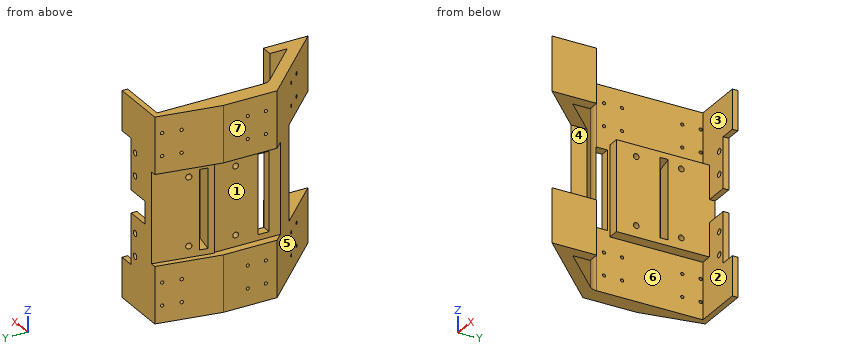
from build123d import *

# Parameters (mm, degrees)
BOSS_EXTRUDE2_DEPTH = 180
SKETCH2_R           = 2.5
CUT_EXTRUDE1_DEPTH  = 180
SKETCH3_W           = 10
SKETCH3_H           = 82.5
CUT_EXTRUDE2_DEPTH  = 35
BOSS_EXTRUDE3_DEPTH = 34
CUT_EXTRUDE3_DEPTH  = 205.147272565
SKETCH6_R           = 2.5
CUT_EXTRUDE4_DEPTH  = 34
CUT_EXTRUDE5_DEPTH  = 5
SKETCH8_W           = 80
SKETCH8_H           = 62.155508182
CUT_EXTRUDE8_DEPTH  = 7
CUT_EXTRUDE9_DEPTH  = 205.147272565
SKETCH11_W          = 10
SKETCH11_H          = 35
BOSS_EXTRUDE4_DEPTH = 5
SKETCH12_W          = 15
SKETCH12_H          = 82.5
CUT_EXTRUDE11_DEPTH = 10
SKETCH10_R          = 1.4
CUT_EXTRUDE10_DEPTH = 18
SKETCH14_R          = 1.4
CUT_EXTRUDE12_DEPTH = 211.50767784
BOSS_EXTRUDE5_DEPTH = 14
SKETCH16_R          = 1.5
CUT_EXTRUDE13_DEPTH = 219.238688301
SKETCH17_W          = 70
SKETCH17_H          = 7
CUT_EXTRUDE14_DEPTH = 210.498896517
SKETCH18_W          = 70
SKETCH18_H          = 10
CUT_EXTRUDE15_DEPTH = 209.444279941
BOSS_EXTRUDE6_DEPTH = 48
FILLET1_R           = 10


# Read off the part's stored shape, not the designer's step: Boss-Extrude2
with BuildPart() as part:
    # Boss-Extrude2 outline → Boss-Extrude2 (new body)
    with BuildSketch(Plane.XY):
        Polygon((-25, 32.5), (-25, -32.5), (-15, -87.5), (25, -87.5), (25, -82.5), (0, -82.5), (0, 82.5), (25, 82.5), (25, 87.5), (-15, 87.5), align=None)
    extrude(amount=BOSS_EXTRUDE2_DEPTH)

    # Sketch2 → Cut-Extrude1 (cut)
    with BuildSketch(Plane(origin=(0, 87.5, 0), x_dir=(1, 0, 0), z_dir=(0, 1, 0))):
        Polygon((25, -35), (21, -35), (21, -80), (0, -80), (0, -100), (21, -100), (21, -145), (25, -145), align=None)
        with Locations(Location((15, -45, 0), (0, 0, 270))):
            Circle(SKETCH2_R)
        with Locations(Location((15, -65, 0), (0, 0, 270))):
            Circle(SKETCH2_R)
        with Locations(Location((15, -115, 0), (0, 0, 270))):
            Circle(SKETCH2_R)
        with Locations(Location((15, -135, 0), (0, 0, 270))):
            Circle(SKETCH2_R)
    extrude(amount=-CUT_EXTRUDE1_DEPTH, mode=Mode.SUBTRACT)

    # Sketch3 → Cut-Extrude2 (cut)
    with BuildSketch(Plane.XY.offset(180)):
        with Locations((-5, 41.25)):
            Rectangle(SKETCH3_W, SKETCH3_H)
    cut_extrude2 = extrude(amount=-CUT_EXTRUDE2_DEPTH, mode=Mode.SUBTRACT)

    # Mirror1: Cut-Extrude2 across plane
    add(cut_extrude2.mirror(Plane.XY.offset(90)), mode=Mode.SUBTRACT)

    # Sketch4 → Boss-Extrude3 (add)
    with BuildSketch(Plane.XY.offset(180)):
        Polygon((-10, 0), (40.247470675, -50.247470675), (40.247470675, -80.498358966), (-25, -15.250888291), align=None)
    boss_extrude3 = extrude(amount=-BOSS_EXTRUDE3_DEPTH)

    # Mirror2: Boss-Extrude3 across plane
    add(boss_extrude3.mirror(Plane.XY.offset(90)))

    # Sketch5 → Cut-Extrude3 (cut, through all)
    with BuildSketch(Plane.XY.offset(180)):
        Polygon((0, 0), (-10, 0), (0, -10), align=None)
        Polygon((0, -40.250888291), (-25, -15.250888291), (-25, -32.5), (-15, -87.5), (25, -87.5), (25, -82.5), (0, -82.5), align=None)
    extrude(amount=-CUT_EXTRUDE3_DEPTH, mode=Mode.SUBTRACT)

    # Sketch6 → Cut-Extrude4 (cut)
    with BuildSketch(Plane(origin=(0, 0, 0), x_dir=(0, 0, -1), z_dir=(1, 0, 0))):
        with Locations(Location((-120, 57.5, 0), (0, 0, 90))):
            Circle(SKETCH6_R)
        with Locations(Location((-60, 57.5, 0), (0, 0, 90))):
            Circle(SKETCH6_R)
        with Locations(Location((-120, 17.5, 0), (0, 0, 90))):
            Circle(SKETCH6_R)
        with Locations(Location((-60, 17.5, 0), (0, 0, 90))):
            Circle(SKETCH6_R)
    extrude(amount=-CUT_EXTRUDE4_DEPTH, mode=Mode.SUBTRACT)

    # Sketch7 → Cut-Extrude5 (cut)
    with BuildSketch(Plane(origin=(-29.92, 5.44, 0), x_dir=(0, 0, 1), z_dir=(-0.9838699100999075, 0.17888543819998307, 0))):
        Polygon((50, 83.405335561), (50, 27.503636123), (130, 27.503636123), (130, 85.782619375), (130, 90.970472455), (50, 90.970472455), align=None)
    extrude(amount=-CUT_EXTRUDE5_DEPTH, mode=Mode.SUBTRACT)

    # Sketch8 → Cut-Extrude8 (cut)
    with BuildSketch(Plane.ZY.offset(25)):
        with Locations((90, 5.923338625)):
            Rectangle(SKETCH8_W, SKETCH8_H)
    extrude(amount=-CUT_EXTRUDE8_DEPTH, mode=Mode.SUBTRACT)

    # Sketch9 → Cut-Extrude9 (cut, through all)
    with BuildSketch(Plane.XY.offset(180)):
        Polygon((-10, 0), (40.247470675, -50.247470675), (40.247470675, -66.356223342), (-10, -16.108752667), align=None)
    extrude(amount=-CUT_EXTRUDE9_DEPTH, mode=Mode.SUBTRACT)

    # Sketch11 → Boss-Extrude4 (add)
    with BuildSketch(Plane(origin=(0, 87.5, 0), x_dir=(1, 0, 0), z_dir=(0, 1, 0))):
        with Locations((30, -17.5)):
            Rectangle(SKETCH11_W, SKETCH11_H)
        with Locations((30, -162.5)):
            Rectangle(SKETCH11_W, SKETCH11_H)
    extrude(amount=-BOSS_EXTRUDE4_DEPTH)

    # Sketch12 → Cut-Extrude11 (cut)
    with BuildSketch(Plane(origin=(0, 0, 0), x_dir=(0, 0, -1), z_dir=(1, 0, 0))):
        with Locations((-137.5, 41.25)):
            Rectangle(SKETCH12_W, SKETCH12_H)
        with Locations((-42.5, 41.25)):
            Rectangle(SKETCH12_W, SKETCH12_H)
    extrude(amount=-CUT_EXTRUDE11_DEPTH, mode=Mode.SUBTRACT)

    # Sketch10 → Cut-Extrude10 (cut)
    with BuildSketch(Plane(origin=(-29.92, 5.44, 0), x_dir=(0, 0, 1), z_dir=(-0.9838699100999075, 0.17888543819998307, 0))):
        with Locations(Location((165, 77.405335561, 0), (0, 0, 270))):
            Circle(SKETCH10_R)
        with Locations(Location((145, 77.405335561, 0), (0, 0, 270))):
            Circle(SKETCH10_R)
        with Locations(Location((145, 61.405335561, 0), (0, 0, 270))):
            Circle(SKETCH10_R)
        with Locations(Location((165, 61.405335561, 0), (0, 0, 270))):
            Circle(SKETCH10_R)
    cut_extrude10 = extrude(amount=-CUT_EXTRUDE10_DEPTH, mode=Mode.SUBTRACT)

    # Mirror3: Cut-Extrude10 across plane
    add(cut_extrude10.mirror(Plane.XY.offset(90)), mode=Mode.SUBTRACT)

    # Sketch14 → Cut-Extrude12 (cut, through all)
    with BuildSketch(Plane.ZY.offset(25)):
        with Locations((165, -5.250888291)):
            Circle(SKETCH14_R)
        with Locations((145, -5.250888291)):
            Circle(SKETCH14_R)
        with Locations((145, 10.749111709)):
            Circle(SKETCH14_R)
        with Locations((165, 10.749111709)):
            Circle(SKETCH14_R)
    cut_extrude12 = extrude(amount=-CUT_EXTRUDE12_DEPTH, mode=Mode.SUBTRACT)

    # Sketch15 → Boss-Extrude5 (add)
    with BuildSketch(Plane(origin=(0, 0, 146), x_dir=(-1, 0, 0), z_dir=(0, 0, -1))):
        Polygon((0, -40.250888291), (0, -26.108752667), (-40.247470675, -66.356223342), (-40.247470675, -80.498358966), align=None)
    boss_extrude5 = extrude(amount=BOSS_EXTRUDE5_DEPTH)

    # Mirror4: Boss-Extrude5 across plane
    add(boss_extrude5.mirror(Plane.XY.offset(90)))

    # Mirror5: Cut-Extrude12 across plane
    add(cut_extrude12.mirror(Plane.XY.offset(90)), mode=Mode.SUBTRACT)

    # Sketch16 → Cut-Extrude13 (cut, through all)
    with BuildSketch(Plane(origin=(-20.125444145, -20.125444145, 0), x_dir=(0, 0, 1), z_dir=(-0.7071067811865476, -0.7071067811865476, 0))):
        with Locations(Location((165, -35.380194939, 0), (0, 0, 270))):
            Circle(SKETCH16_R)
        with Locations(Location((145, -35.380194939, 0), (0, 0, 270))):
            Circle(SKETCH16_R)
        with Locations(Location((145, -51.380194939, 0), (0, 0, 270))):
            Circle(SKETCH16_R)
        with Locations(Location((165, -51.380194939, 0), (0, 0, 270))):
            Circle(SKETCH16_R)
    cut_extrude13 = extrude(amount=-CUT_EXTRUDE13_DEPTH, mode=Mode.SUBTRACT)

    # Mirror6: Cut-Extrude13 across plane
    add(cut_extrude13.mirror(Plane.XY.offset(90)), mode=Mode.SUBTRACT)

    # Sketch17 → Cut-Extrude14 (cut, through all)
    with BuildSketch(Plane(origin=(-25.00065045, 4.545572809, 0), x_dir=(0, 0, 1), z_dir=(-0.9838699100999075, 0.17888543819998304, 0))):
        with Locations((90, 41.684323876)):
            Rectangle(SKETCH17_W, SKETCH17_H)
    extrude(amount=-CUT_EXTRUDE14_DEPTH, mode=Mode.SUBTRACT)

    # Sketch18 → Cut-Extrude15 (cut, through all)
    with BuildSketch(Plane.ZY.offset(18)):
        with Locations((90, -7.250888291)):
            Rectangle(SKETCH18_W, SKETCH18_H)
    extrude(amount=-CUT_EXTRUDE15_DEPTH, mode=Mode.SUBTRACT)

    # Sketch19 → Boss-Extrude6 (add)
    with BuildSketch(Plane.XY.offset(180)):
        Polygon((30.247470675, -56.356223342), (40.247470675, -66.356223342), (40.247470675, -40.856223342), (30.247470675, -40.856223342), align=None)
    boss_extrude6 = extrude(amount=-BOSS_EXTRUDE6_DEPTH)

    # Mirror7: Boss-Extrude6 across plane
    add(boss_extrude6.mirror(Plane.XY.offset(90)))

    # Fillet1
    # the kernel refuses this fillet: 10 mm, written as the material it adds along each edge
    with BuildSketch(Plane(origin=(-10, -16.108752667, 180), x_dir=(0, 1, 0), z_dir=(0, 0, -1))) as fillet1_piece_1_section:
        with BuildLine():
            CenterArc((FILLET1_R * 0.414213562373, FILLET1_R), FILLET1_R, 225, 45)
            Line((-FILLET1_R * 0.292893218813, FILLET1_R * 0.292893218813), (0, 0))
            Line((0, 0), (FILLET1_R * 0.414213562373, 0))
        make_face()
    fillet1_piece_1 = extrude(amount=180, mode=Mode.PRIVATE)
    fillet1_piece_1 = split(fillet1_piece_1, bisect_by=Plane(origin=(-10.099322896, -12.109228126, 125), z_dir=(0, 0, 1)), keep=Keep.TOP, mode=Mode.PRIVATE)
    fillet1_piece_1 = split(fillet1_piece_1, bisect_by=Plane(origin=(-10.099322896, -12.250888291, 152.5), z_dir=(0, 1, 0)), keep=Keep.TOP, mode=Mode.PRIVATE)
    add(fillet1_piece_1)
    with BuildSketch(Plane(origin=(-10, -16.108752667, 180), x_dir=(0, 1, 0), z_dir=(0, 0, -1))) as fillet1_piece_2_section:
        with BuildLine():
            CenterArc((FILLET1_R * 0.414213562373, FILLET1_R), FILLET1_R, 225, 45)
            Line((-FILLET1_R * 0.292893218813, FILLET1_R * 0.292893218813), (0, 0))
            Line((0, 0), (FILLET1_R * 0.414213562373, 0))
        make_face()
    fillet1_piece_2 = extrude(amount=180, mode=Mode.PRIVATE)
    fillet1_piece_2 = split(fillet1_piece_2, bisect_by=Plane(origin=(-9.370999607, -15.909597181, 125), z_dir=(0, 0, 1)), keep=Keep.TOP, mode=Mode.PRIVATE)
    fillet1_piece_2 = split(fillet1_piece_2, bisect_by=Plane(origin=(-9.370999607, -12.250888291, 152.5), z_dir=(0, -1, 0)), keep=Keep.TOP, mode=Mode.PRIVATE)
    add(fillet1_piece_2)
    with BuildSketch(Plane(origin=(-10, -16.108752667, 180), x_dir=(0, 1, 0), z_dir=(0, 0, -1))) as fillet1_piece_3_section:
        with BuildLine():
            CenterArc((FILLET1_R * 0.414213562373, FILLET1_R), FILLET1_R, 225, 45)
            Line((-FILLET1_R * 0.292893218813, FILLET1_R * 0.292893218813), (0, 0))
            Line((0, 0), (FILLET1_R * 0.414213562373, 0))
        make_face()
    fillet1_piece_3 = extrude(amount=180, mode=Mode.PRIVATE)
    fillet1_piece_3 = split(fillet1_piece_3, bisect_by=Plane(origin=(-9.370999607, -15.909597181, 125), z_dir=(0, 0, -1)), keep=Keep.TOP, mode=Mode.PRIVATE)
    fillet1_piece_3 = split(fillet1_piece_3, bisect_by=Plane(origin=(-9.370999607, -12.250888291, 90), z_dir=(0, -1, 0)), keep=Keep.TOP, mode=Mode.PRIVATE)
    fillet1_piece_3 = split(fillet1_piece_3, bisect_by=Plane(origin=(-9.370999607, -15.909597181, 55), z_dir=(0, 0, 1)), keep=Keep.TOP, mode=Mode.PRIVATE)
    add(fillet1_piece_3)
    with BuildSketch(Plane(origin=(-10, -16.108752667, 180), x_dir=(0, 1, 0), z_dir=(0, 0, -1))) as fillet1_piece_4_section:
        with BuildLine():
            CenterArc((FILLET1_R * 0.414213562373, FILLET1_R), FILLET1_R, 225, 45)
            Line((-FILLET1_R * 0.292893218813, FILLET1_R * 0.292893218813), (0, 0))
            Line((0, 0), (FILLET1_R * 0.414213562373, 0))
        make_face()
    fillet1_piece_4 = extrude(amount=180, mode=Mode.PRIVATE)
    fillet1_piece_4 = split(fillet1_piece_4, bisect_by=Plane(origin=(-10.099322896, -12.250888291, 27.5), z_dir=(0, 1, 0)), keep=Keep.TOP, mode=Mode.PRIVATE)
    fillet1_piece_4 = split(fillet1_piece_4, bisect_by=Plane(origin=(-10.099322896, -12.109228126, 55), z_dir=(0, 0, -1)), keep=Keep.TOP, mode=Mode.PRIVATE)
    add(fillet1_piece_4)
    with BuildSketch(Plane(origin=(-10, -16.108752667, 180), x_dir=(0, 1, 0), z_dir=(0, 0, -1))) as fillet1_piece_5_section:
        with BuildLine():
            CenterArc((FILLET1_R * 0.414213562373, FILLET1_R), FILLET1_R, 225, 45)
            Line((-FILLET1_R * 0.292893218813, FILLET1_R * 0.292893218813), (0, 0))
            Line((0, 0), (FILLET1_R * 0.414213562373, 0))
        make_face()
    fillet1_piece_5 = extrude(amount=180, mode=Mode.PRIVATE)
    fillet1_piece_5 = split(fillet1_piece_5, bisect_by=Plane(origin=(-9.370999607, -12.250888291, 27.5), z_dir=(0, -1, 0)), keep=Keep.TOP, mode=Mode.PRIVATE)
    fillet1_piece_5 = split(fillet1_piece_5, bisect_by=Plane(origin=(-9.370999607, -15.909597181, 55), z_dir=(0, 0, -1)), keep=Keep.TOP, mode=Mode.PRIVATE)
    add(fillet1_piece_5)


solid = part.part
Read the model definition and answer for the solid it produces. Units are mm, in the model's axes. Face numbers are marked on the shaded views. A direction names the side the tool comes from. Coordinates: 2 decimals unless noted, no trailing zeros. Loops run counter-clockwise (first coordinate to the right, second up) from the corner with the lowest first, then second, coordinate; pieces in that order, holes last.
Q1. The mould has two halves that part along Y. Classify the marked faces 5, 6 and 7: +Y half, -Y half, draft (parallel to the pull), parting line (faces both ways), or undercut.
Q2. Consider probe 1 along Z at (x, y) = (-5.25, 57.5); probe 2 along Z at (x, y) = (-11, 41); probe 3 along Y at (x, z) = (23, 23.5). Determine where each line is inside the solid, lowest interval first.
Q3. Each of these flat-tipped pins is pushed along its axis until it touches: pin 1 Ø10 at (y, z) = (60.5, 92.5) entering from +X; pin 2 Ø4 at (x, z) = (-3, 44) entering from -Y; pin 3 Ø2 at (y, z) = (-5.25, 165) entering from -X; pin 4 Ø2 at (y, z) = (-15, 125.5) entering from -X. Where does it stop, or does it pass through?
Q4. The part is cut by section A-A on z = 65. Write down the section's boundary in (x, y), and give its area (3 significant figures).
Q5. The part is cut by section D-D on y = 57.5. Write down the section's boundary in (x, z), and give its area (3 significant figures).
Q6. The part is cut by section B-B on z = 45. Write down the section's boundary in (x, y), and give its area (3 significant figures).
Q7. Which of the six approach directions +Z, -Z, +X, -X, +Y, -Y give full straight-line access (tool end or side, diameter ignored) to the marked faces 1, 2, 3 and 4?
Q8. The part is cut by section C-C on y = -68. Write down the section's boundary in (x, z), and give its area (3 significant figures).
Results below:
1. face 5: -Y half
1. face 6: undercut
1. face 7: draft
2. probe 1: z = 50 to 57.5, 62.5 to 117.5, 122.5 to 130
2. probe 2: z = 0 to 55, 125 to 180
2. probe 3: y = -63.25 to -49.11, 82.5 to 87.5
3. pin 1: stops at x = 0
3. pin 2: stops at y = -39.25
3. pin 3: passes through
3. pin 4: stops at x = -18
4. outline: (-19.1, 37) - (-18, 37) - (-18, -2.25) - (-10, -2.25) - (-10, 0) - (0, 0) - (0, 38.81) - (-18.17, 42.11) - close; (-18, -22.25) - (0, -40.25) - (0, -26.11) - (-7.07, -19.04) arc R10 cw to (-10, -12.25) - (-18, -12.25) - close; (-16.92, 49) - (0, 45.93) - (0, 82.5) - (12.5, 82.5) - (12.5, 87.5) - (-9.92, 87.5) - close; (17.5, 82.5) - (21, 82.5) - (21, 87.5) - (17.5, 87.5) - close
4. area: 1,630 mm2
5. outline: (-20.45, 0) - (-10, 0) - (-10, 50) - (0, 50) - (0, 57.5) - (-15.37, 57.5) - (-15.37, 50) - (-20.45, 50) - close; (-20.45, 130) - (-15.37, 130) - (-15.37, 122.5) - (0, 122.5) - (0, 130) - (-10, 130) - (-10, 180) - (-20.45, 180) - close; (-15.37, 62.5) - (0, 62.5) - (0, 117.5) - (-15.37, 117.5) - close
5. area: 2,120 mm2
6. outline: (-25, -15.25) - (40.25, -80.5) - (40.25, -40.86) - (30.25, -40.86) - (30.25, -56.36) - (-7.07, -19.04) arc R10 cw to (-10, -11.97) - (-10, 82.5) - (12.5, 82.5) - (12.5, 87.5) - (-15, 87.5) - (-25, 32.5) - close; (17.5, 82.5) - (21, 82.5) - (21, 87.5) - (17.5, 87.5) - close
6. area: 2,430 mm2
7. face 1: -X, -Y
7. face 2: -Z, +X
7. face 3: +Z, +X
7. face 4: +X, -Y
8. outline: (27.75, 0) - (40.25, 0) - (40.25, 48) - (27.75, 48) - close; (27.75, 132) - (40.25, 132) - (40.25, 180) - (27.75, 180) - close
8. area: 1,200 mm2
